from build123d import *

# Parameters (mm, degrees)
ESQUISSE1_R        = 6
ESQUISSE1_R_2      = 5
BOSS_EXTRU_1_DEPTH = 9
ESQUISSE2_R        = 7.5
ESQUISSE2_R_2      = 5
BOSS_EXTRU_2_DEPTH = 7
ESQUISSE3_R        = 8.5
ESQUISSE3_R_2      = 5
BOSS_EXTRU_3_DEPTH = 2
ESQUISSE4_R        = 7.5
ESQUISSE4_R_2      = 5
BOSS_EXTRU_4_DEPTH = 13
ESQUISSE5_R        = 6
ESQUISSE5_R_2      = 5
BOSS_EXTRU_5_DEPTH = 20


with BuildPart() as part:
    # Esquisse1 → Boss.-Extru.1 (new body)
    with BuildSketch(Plane(origin=(0, 0, 0), x_dir=(1, 0, 0), z_dir=(0, 1, 0))):
        Circle(ESQUISSE1_R)
        Circle(ESQUISSE1_R_2, mode=Mode.SUBTRACT)
    extrude(amount=BOSS_EXTRU_1_DEPTH)

    # Esquisse2 → Boss.-Extru.2 (add)
    with BuildSketch(Plane(origin=(0, 9, 0), x_dir=(1, 0, 0), z_dir=(0, 1, 0))):
        Circle(ESQUISSE2_R)
        Circle(ESQUISSE2_R_2, mode=Mode.SUBTRACT)
    extrude(amount=BOSS_EXTRU_2_DEPTH)

    # Esquisse3 → Boss.-Extru.3 (add)
    with BuildSketch(Plane(origin=(0, 16, 0), x_dir=(1, 0, 0), z_dir=(0, 1, 0))):
        Circle(ESQUISSE3_R)
        Circle(ESQUISSE3_R_2, mode=Mode.SUBTRACT)
    extrude(amount=BOSS_EXTRU_3_DEPTH)

    # Esquisse4 → Boss.-Extru.4 (add)
    with BuildSketch(Plane(origin=(0, 18, 0), x_dir=(1, 0, 0), z_dir=(0, 1, 0))):
        Circle(ESQUISSE4_R)
        Circle(ESQUISSE4_R_2, mode=Mode.SUBTRACT)
    extrude(amount=BOSS_EXTRU_4_DEPTH)

    # Esquisse5 → Boss.-Extru.5 (add)
    with BuildSketch(Plane(origin=(0, 31, 0), x_dir=(1, 0, 0), z_dir=(0, 1, 0))):
        Circle(ESQUISSE5_R)
        Circle(ESQUISSE5_R_2, mode=Mode.SUBTRACT)
    extrude(amount=BOSS_EXTRU_5_DEPTH)


solid = part.part
Build history of the part. All positions in model axes, mm. A direction names the side the tool comes from. Round coordinates to 2 decimals unless told otherwise and drop trailing zeros. Loops run counter-clockwise (first coordinate to the right, second up) from the corner with the lowest first, then second, coordinate; pieces in that order, holes last. Notation, with made-up numbers: (3.25, 9) -> (59.25, 9) arc R26 cw to (59.25, 43) -> close; hole circle Ø2 at (57.25, 51.5). An arc over 180 degrees is marked (long way). One line per item, written item: value. Start each with the question number.
Q1. Cut at D-D on x = 5.5. List the corners of the cut face in (y, z).
Q2. Cut at A-A on x = 0. List the corners of the cut face in (y, z).
Q3. Cut at C-C on y = 47.5. List the corners of the cut face in (x, z).
Q4. 3-axis set-ups, long thin cutter, end or side, ignore diameter. For faces 4 (the face through (-7.493, 12.451, -0.33)), 5 (the face through (-4, 0, -4)), 6 (the face through (-6, 41, 0)): which of +Z, -Z, +X, -X, +Y, -Y reach the whole face in a straight line?
Q5. Two-plate mould, pull along Z, no slides. Class faces 1 (the face through (-4, 51, -4)), 2 (the face through (-1.08, 25.14, 4.88)), 3 (the face through (-7.493, 24.409, -0.33)): released by +Z, released by -Z, zero draft, split by the parting line, or undercut.
Q6. Drop flat-ended pins along their axis: pin 1 Ø3 at (y, z) = (13.5, -1) entering from +X; pin 2 Ø3 at (y, z) = (40, -3) entering from +X; pin 3 Ø1 at (y, z) = (27, 3) entering from +X. Give the stop position or say it passes through.
Q7. Cut at B-B on z = 0. List the corners of the cut face in (x, y).
Q8. Probe line 1 along Z through (x, y) = (0, 11); line 2 along Z through (x, y) = (0, 38.5). List the from-to ranges inside material, lowest first.
Computed:
1. outline: (0, -2.4) -> (9, -2.4) -> (9, -5.1) -> (16, -5.1) -> (16, -6.48) -> (18, -6.48) -> (18, -5.1) -> (31, -5.1) -> (31, -2.4) -> (51, -2.4) -> (51, 2.4) -> (31, 2.4) -> (31, 5.1) -> (18, 5.1) -> (18, 6.48) -> (16, 6.48) -> (16, 5.1) -> (9, 5.1) -> (9, 2.4) -> (0, 2.4) -> close
2. outline: (0, -6) -> (9, -6) -> (9, -7.5) -> (16, -7.5) -> (16, -8.5) -> (18, -8.5) -> (18, -7.5) -> (31, -7.5) -> (31, -6) -> (51, -6) -> (51, -5) -> (0, -5) -> close; (0, 5) -> (51, 5) -> (51, 6) -> (31, 6) -> (31, 7.5) -> (18, 7.5) -> (18, 8.5) -> (16, 8.5) -> (16, 7.5) -> (9, 7.5) -> (9, 6) -> (0, 6) -> close
3. outline: circle Ø12 at (0, 0); hole circle Ø10 at (0, 0)
4. face 4: -Y
4. face 5: +Z, -Z, +X, -X, -Y
4. face 6: +Y
5. face 1: zero draft
5. face 2: undercut
5. face 3: split by the parting line
6. pin 1: x = 7.5
6. pin 2: x = 5.81
6. pin 3: x = 7.07
7. outline: (-8.5, 16) -> (-7.5, 16) -> (-7.5, 9) -> (-6, 9) -> (-6, 0) -> (-5, 0) -> (-5, 51) -> (-6, 51) -> (-6, 31) -> (-7.5, 31) -> (-7.5, 18) -> (-8.5, 18) -> close; (5, 0) -> (6, 0) -> (6, 9) -> (7.5, 9) -> (7.5, 16) -> (8.5, 16) -> (8.5, 18) -> (7.5, 18) -> (7.5, 31) -> (6, 31) -> (6, 51) -> (5, 51) -> close
8. line 1: -7.5 to -5, 5 to 7.5
8. line 2: -6 to -5, 5 to 6
